```python
from build123d import *

# Parameters (mm, degrees)
SKETCH1_W               = 60
SKETCH1_H               = 60
BOSS_EXTRUDE1_DEPTH     = 10
SKETCH6_R               = 8.5
SKETCH7_RX              = 8.5
SKETCH7_RY              = 6.01040764
SKETCH8_W               = 60
SKETCH8_H               = 60
SKETCH8_RX              = 8.5
SKETCH8_RY              = 6.01040764
BOSS_EXTRUDE2_DEPTH     = 30
SKETCH9_R               = 3
CUT_EXTRUDE1_DEPTH      = 41
SKETCH10_R              = 3
CUT_EXTRUDE2_DEPTH      = 61
SKETCH11_W              = 16.5
SKETCH11_H              = 21
CUT_EXTRUDE3_DEPTH      = 12.5
SKETCH12_W              = 16.5
SKETCH12_H              = 6
CUT_EXTRUDE4_DEPTH      = 8.5
SKETCH13_W              = 4
SKETCH13_H              = 3
CUT_EXTRUDE5_DEPTH      = 18.5
FILLET1_R               = 10
SKETCH14_W              = 18
SKETCH14_H              = 1
CUT_EXTRUDE7_DEPTH      = 20
CUT_EXTRUDE7_DEPTH_BACK = 14.142136


with BuildPart() as part:
    # Sketch1 → Boss-Extrude1 (new body)
    with BuildSketch(Plane(origin=(0, 0, 0), x_dir=(1, 0, 0), z_dir=(0, 1, 0))):
        Rectangle(SKETCH1_W, SKETCH1_H)
    extrude(amount=BOSS_EXTRUDE1_DEPTH)

    # Sketch6 → Loft1 section 0
    with BuildSketch(Plane(origin=(15, 15, 0), x_dir=(0, 0, -1), z_dir=(0.707106781, 0.707106781, 0))):
        with Locations((0, 21.213203436)):
            Circle(SKETCH6_R)
    # Sketch7 → Loft1 section 1
    with BuildSketch(Plane(origin=(0, 10, 0), x_dir=(1, 0, 0), z_dir=(0, 1, 0))):
        with Locations(Location((0, 0), (0, 0, 90))):
            Ellipse(SKETCH7_RX, SKETCH7_RY)
    loft()

    # Sketch8 → Boss-Extrude2 (add)
    with BuildSketch(Plane(origin=(0, 10, 0), x_dir=(1, 0, 0), z_dir=(0, 1, 0))):
        Rectangle(SKETCH8_W, SKETCH8_H)
        with Locations(Location((0, 0), (0, 0, 90))):
            Ellipse(SKETCH8_RX, SKETCH8_RY, mode=Mode.SUBTRACT)
    extrude(amount=BOSS_EXTRUDE2_DEPTH)

    # Sketch9 → Cut-Extrude1 (cut, through all)
    with BuildSketch(Plane(origin=(0, 40, 0), x_dir=(1, 0, 0), z_dir=(0, 1, 0))):
        Circle(SKETCH9_R)
    extrude(amount=-CUT_EXTRUDE1_DEPTH, mode=Mode.SUBTRACT)

    # Sketch10 → Cut-Extrude2 (cut, through all)
    with BuildSketch(Plane(origin=(30, 0, 0), x_dir=(0, 0, -1), z_dir=(1, 0, 0))):
        with Locations((0, 30)):
            Circle(SKETCH10_R)
    extrude(amount=-CUT_EXTRUDE2_DEPTH, mode=Mode.SUBTRACT)

    # Sketch11 → Cut-Extrude3 (cut)
    with BuildSketch(Plane(origin=(30, 0, 0), x_dir=(0, 0, -1), z_dir=(1, 0, 0))):
        with Locations((0, 29.5)):
            Rectangle(SKETCH11_W, SKETCH11_H)
    extrude(amount=-CUT_EXTRUDE3_DEPTH, mode=Mode.SUBTRACT)

    # Sketch12 → Cut-Extrude4 (cut)
    with BuildSketch(Plane(origin=(17.5, 0, 0), x_dir=(0, 0, -1), z_dir=(1, 0, 0))):
        with Locations((0, 22)):
            Rectangle(SKETCH12_W, SKETCH12_H)
    extrude(amount=-CUT_EXTRUDE4_DEPTH, mode=Mode.SUBTRACT)

    # Sketch13 → Cut-Extrude5 (cut)
    with BuildSketch(Plane(origin=(9, 0, 0), x_dir=(0, 0, -1), z_dir=(1, 0, 0))):
        with Locations((0, 17.5)):
            Rectangle(SKETCH13_W, SKETCH13_H)
    extrude(amount=CUT_EXTRUDE5_DEPTH, mode=Mode.SUBTRACT)

    # Fillet1
    fillet1_edges = [part.edges().sort_by_distance(p)[0] for p in [
        (23.75, 40, 8.25),
        (23.75, 40, -8.25),
    ]]
    fillet(fillet1_edges, radius=FILLET1_R)

    # Sketch14 → Cut-Extrude7 (cut, two sides)
    with BuildSketch(Plane(origin=(-25, 25, 0), x_dir=(0, 0, 1), z_dir=(-0.707106781, 0.707106781, 0))) as cut_extrude7_sk:
        with Locations((0, 21.713203436)):
            Rectangle(SKETCH14_W, SKETCH14_H)
    extrude(amount=CUT_EXTRUDE7_DEPTH, mode=Mode.SUBTRACT)
    extrude(cut_extrude7_sk.sketch, amount=-CUT_EXTRUDE7_DEPTH_BACK, mode=Mode.SUBTRACT)


solid = part.part
```
Could you check a few things on this model? Use its own coordinates, in mm. A direction names the side the tool comes from. Round coordinates to 2 decimals unless told otherwise and drop trailing zeros. Loops run counter-clockwise (first coordinate to the right, second up) from the corner with the lowest first, then second, coordinate; pieces in that order, holes last. Notation, with made-up numbers: M 87,79.5 L 98,79.5 A20 ccw 98,92.5 Z; hole C 12,-17 d10. An arc over 180 degrees is marked long. Answer as CSV lines item,"result".
1) Imagine slicing it at B-B on x = 26. List the corners of the cut face in (y, z) for me, and give its area (3 significant figures).
From the geometry:
outline,"M 0,-30 L 40,-30 L 40,-18.25 A10 ccw 30,-8.25 L 19,-8.25 L 19,-2 L 16,-2 L 16,2 L 19,2 L 19,8.25 L 30,8.25 A10 ccw 40,18.25 L 40,30 L 0,30 Z"
area,"2,000 mm^2"
2) Which directions (+Z, -Z, +X, -X, +Y, -Y) give clear straight access to the entire face, cutting with the end or side of a thin tool? Please do faces 1 (the flat face through (27.5, 18, 0)), 2 (the flat face through (22, 23, 8.25)), 3 (the flat face through (18, 16, 0)).
From the geometry:
face 1,"+Y"
face 2,"+X"
face 3,"none"
3) For pin 1 Ø1 at (x, z) = (18.5, 12) entering from +Y, with a flat end and sliding along its axis, tell me the tip position at first contact or that it passes through.
From the geometry:
pin 1,"y = 38.18"
4) Imagine slicing it at C-C on z = 1. Count the separate pieces of the cut face and the enclosed holes in it, and give its area (3 significant figures).
From the geometry:
separate pieces,"5"
enclosed holes,"0"
area,"1,520 mm^2"
5) We'd pull the mould along Y, two halves only. Please class faces 4 (the cylindrical face through (23.66, 37.15, 11.26)), 5 (the flat face through (20, 19, -4)), 6 (the flat face through (0, 20, -30)): released by +Y, released by -Y, zero draft, split by the parting line, or undercut.
From the geometry:
face 4,"released by +Y"
face 5,"undercut"
face 6,"zero draft"
6) Imagine slicing it at A-A on x = 13. List the corners of the cut face in (y, z) for me, and give its area (3 significant figures).
From the geometry:
outline,"M 0,-30 L 40,-30 L 40,30 L 0,30 Z; hole M 16,-2 L 19,-2 L 19,-8.25 L 25,-8.25 L 25,8.25 L 19,8.25 L 19,2 L 16,2 Z; hole C 30,0 d6"
area,"2,260 mm^2"
7) If I drill on probe 1 along Y at (x, z) = (14.25, 0); probe 2 along Z at (x, y) = (-20.5, 30), over which ranges is the centre line in solid material (lowest first)?
From the geometry:
probe 1,"0 to 16, 25 to 27, 33 to 40"
probe 2,"-30 to -3, 3 to 30"
